from build123d import *

# Parameters (mm, degrees)
SKETCH_3_W          = 5
SKETCH_3_H          = 5
EXTRUDE_2_DEPTH     = 1
SKETCH_4_R          = 3.535533906
EXTRUDE_3_DEPTH     = 1
SKETCH_5_R          = 2.5
EXTRUDE_4_DEPTH     = 9.3
CUT_EXTRUDE_1_REACH = 15.377
SKETCH_7_R          = 0.9


with BuildPart() as part:
    # 草图3 → 凸台-拉伸2 (new body)
    with BuildSketch(Plane(origin=(0, 0, 0), x_dir=(1, 0, 0), z_dir=(0, 1, 0))):
        with Locations((2.5, 2.5)):
            Rectangle(SKETCH_3_W, SKETCH_3_H)
    extrude(amount=EXTRUDE_2_DEPTH)

    # 草图4 → 凸台-拉伸3 (add)
    with BuildSketch(Plane.XZ):
        with Locations(Location((2.5, -2.5, 0), (0, 0, 45))):
            Circle(SKETCH_4_R)
    extrude(amount=EXTRUDE_3_DEPTH)

    # 草图5 → 凸台-拉伸4 (add)
    with BuildSketch(Plane(origin=(0, 1, 0), x_dir=(1, 0, 0), z_dir=(0, 1, 0))):
        with Locations(Location((2.5, 2.5, 0), (0, 0, 270))):
            Circle(SKETCH_5_R)
    extrude(amount=EXTRUDE_4_DEPTH)

    # 草图7 → 切除-拉伸1 (cut, up to next)
    with BuildSketch(Plane(origin=(0, 0, -5), x_dir=(-1, 0, 0), z_dir=(0, 0, -1)), mode=Mode.PRIVATE) as cut_extrude_1_sk1:
        with Locations((-2.5, 8.3)):
            Circle(SKETCH_7_R)
    cut_extrude_1_tool1 = extrude(cut_extrude_1_sk1.sketch, amount=-CUT_EXTRUDE_1_REACH, mode=Mode.PRIVATE) & part.part
    add(cut_extrude_1_tool1.solids().sort_by_distance((2.5, 8.3, -5))[0], mode=Mode.SUBTRACT)


solid = part.part
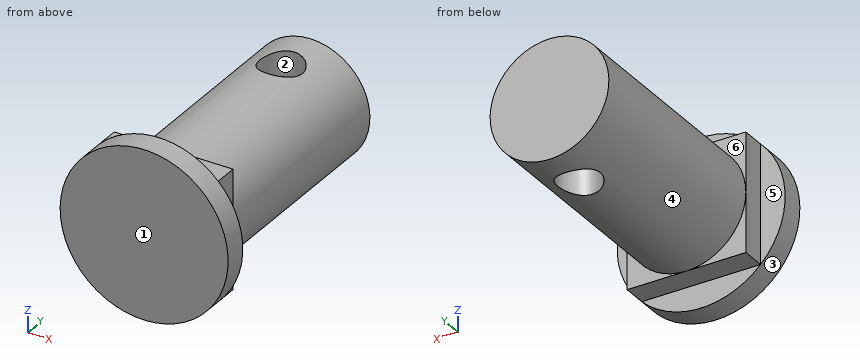
CAD build for the part. Positions are in the model's coordinates, mm. Face numbers are marked on the shaded views. A direction names the side the tool comes from. Round coordinates to 2 decimals unless told otherwise and drop trailing zeros. Loops run counter-clockwise (first coordinate to the right, second up) from the corner with the lowest first, then second, coordinate; pieces in that order, holes last.
(1) Wall check: line 1 along Y through (x, z) = (2.5, -2.6); line 2 along X through (y, z) = (0.75, -2.5); line 3 along X through (y, z) = (8.3, -3.3). Give the ranges that are in metal, low to high.
(2) Drop flat-ended pins along their axis: pin 1 (2 mm diameter, centred on x = 4, y = 4.5, fed in from -Z); pin 2 (1.6 mm diameter, centred on x = 2.5, y = 8.3, fed in from -Z); pin 3 (0.5 mm diameter, centred on x = 2, y = 0.5, fed in from -Z); pin 4 (0.8 mm diameter, centred on x = 3.5, z = 1, fed in from +Y). Give the stop position or say it passes through.
(3) Which spindle directions (+Z, -Z, +X, -X, +Y, -Y) get a long thin tool onto all of the face, cutting with end or side? Do the marked faces 4, 5 and 6. Say none if no direction does.
(4) Cut at D-D (y = 8.3). Give the cut face in (x, z).
(5) Cut at C-C (x = 3.75). Give the cut face in (y, z).
(6) Two-plate mould, pull along X, no slides. Class the marked faces 1, 2 and 3: +X half, -X half, draft (parallel to the pull), parting line (faces both ways), or undercut.
(7) Cut at B-B (y = 0.5). Give the cut face in (x, z).
(8) Cut at A-A (z = -1.5). Give the cut face in (x, y).
Findings below:
1. line 1: y = -1 to 7.4, 9.2 to 10.3
1. line 2: x = 0 to 5
1. line 3: x = 0.13 to 1.6, 3.4 to 4.87
2. pin 1: stops at z = -4.95
2. pin 2: passes through
2. pin 3: stops at z = -5
2. pin 4: stops at y = 0
3. face 4: +Y
3. face 5: +Z, -Z, -X, +Y
3. face 6: +Z, -X, +Y
4. outline: (1.6, -4.83) - (1.6, -0.17) arc R2.5 ccw to start; (3.4, -4.83) arc R2.5 ccw to (3.4, -0.17) - close
5. outline: (-1, -5.81) - (0, -5.81) - (0, -5) - (1, -5) - (1, -4.67) - (10.3, -4.67) - (10.3, -0.33) - (1, -0.33) - (1, 0) - (0, 0) - (0, 0.81) - (-1, 0.81) - close
6. face 1: draft
6. face 2: undercut
6. face 3: parting line
7. outline: (0, -5) - (5, -5) - (5, 0) - (0, 0) - close
8. outline: (-0.89, -1) - (5.89, -1) - (5.89, 0) - (5, 0) - (5, 1) - (4.79, 1) - (4.79, 10.3) - (0.21, 10.3) - (0.21, 1) - (0, 1) - (0, 0) - (-0.89, 0) - close; hole circle Ø1.8 at (2.5, 8.3)
